Can you work these out from the model? Positions are in its coordinate system, mm. A direction names the side the tool comes from. Round coordinates to 2 decimals unless told otherwise and drop trailing zeros. Order: outer loops, then holes, each group sorted by start corner. A loop starts at its lowest first (then second) coordinate and runs counter-clockwise, first axis right, second up. Notation, with made-up numbers: M 33,84.5 L 70,84.5 A26 cw 70,119.5 Z; hole C 55.5,1.25 d4. An arc over 180 degrees is marked long. One line per question, with ' | ' between items.
```python
from build123d import *

# Parameters (mm, degrees)
CUT_EXTRUDE_1_REACH             = 31.394
SKETCH_3_R                      = 2
CUT_EXTRUDE_1_DIRECTION_2_DEPTH = 30.393876913


with BuildPart() as part:
    # 草图2 → 旋转1 (revolve)
    with BuildSketch(Plane.XY):
        Polygon((0, 0), (-20, 0), (-20, 2), (-17.5, 2), (-17.5, 8), (0, 8), align=None)
    revolve(axis=Axis((0, 8, 0), (0, -1, 0)))

    # 草图3 → 切除-拉伸1 (cut, up to next)
    with BuildSketch(Plane(origin=(0, 8, 0), x_dir=(1, 0, 0), z_dir=(0, 1, 0)), mode=Mode.PRIVATE) as cut_extrude_1_sk1:
        with Locations((0, 15)):
            Circle(SKETCH_3_R)
    cut_extrude_1_tool1 = extrude(cut_extrude_1_sk1.sketch, amount=-CUT_EXTRUDE_1_REACH, mode=Mode.PRIVATE) & part.part
    # 草图3 → 切除-拉伸1 (cut, up to next)
    with BuildSketch(Plane(origin=(0, 8, 0), x_dir=(1, 0, 0), z_dir=(0, 1, 0)), mode=Mode.PRIVATE) as cut_extrude_1_sk2:
        with Locations((15, 0)):
            Circle(SKETCH_3_R)
    cut_extrude_1_tool2 = extrude(cut_extrude_1_sk2.sketch, amount=-CUT_EXTRUDE_1_REACH, mode=Mode.PRIVATE) & part.part
    # 草图3 → 切除-拉伸1 (cut, up to next)
    with BuildSketch(Plane(origin=(0, 8, 0), x_dir=(1, 0, 0), z_dir=(0, 1, 0)), mode=Mode.PRIVATE) as cut_extrude_1_sk3:
        with Locations((0, -15)):
            Circle(SKETCH_3_R)
    cut_extrude_1_tool3 = extrude(cut_extrude_1_sk3.sketch, amount=-CUT_EXTRUDE_1_REACH, mode=Mode.PRIVATE) & part.part
    # 草图3 → 切除-拉伸1 (cut, up to next)
    with BuildSketch(Plane(origin=(0, 8, 0), x_dir=(1, 0, 0), z_dir=(0, 1, 0)), mode=Mode.PRIVATE) as cut_extrude_1_sk4:
        with Locations((-15, 0)):
            Circle(SKETCH_3_R)
    cut_extrude_1_tool4 = extrude(cut_extrude_1_sk4.sketch, amount=-CUT_EXTRUDE_1_REACH, mode=Mode.PRIVATE) & part.part
    add(cut_extrude_1_tool1.solids().sort_by_distance((0, 8, -15))[0], mode=Mode.SUBTRACT)
    add(cut_extrude_1_tool2.solids().sort_by_distance((15, 8, 0))[0], mode=Mode.SUBTRACT)
    add(cut_extrude_1_tool3.solids().sort_by_distance((0, 8, 15))[0], mode=Mode.SUBTRACT)
    add(cut_extrude_1_tool4.solids().sort_by_distance((-15, 8, 0))[0], mode=Mode.SUBTRACT)

    # 草图3 → 切除-拉伸1 direction 2 (cut)
    with BuildSketch(Plane(origin=(0, 8, 0), x_dir=(1, 0, 0), z_dir=(0, 1, 0))):
        with Locations((0, 15)):
            Circle(SKETCH_3_R)
        with Locations((15, 0)):
            Circle(SKETCH_3_R)
        with Locations((0, -15)):
            Circle(SKETCH_3_R)
        with Locations((-15, 0)):
            Circle(SKETCH_3_R)
    extrude(amount=CUT_EXTRUDE_1_DIRECTION_2_DEPTH, mode=Mode.SUBTRACT)


solid = part.part
```
(1) Will these pins go through, and if not, where does the flat tip stop? pin 1 Ø1 at (x, y) = (-3.5, 4.5) entering from +Z; pin 2 Ø1.5 at (x, y) = (-15, 2.5) entering from -Z; pin 3 Ø2 at (x, y) = (16, 4.5) entering from +Z.
Final values:
pin 1: z = 17.24 | pin 2: z = -13.84 | pin 3: z = 9.01
(2) If we section it at B-B on x = 0: Please give me the cut outline in (y, z).
Final values:
outline: M 0,-20 L 2,-20 L 2,-17.5 L 8,-17.5 L 8,-17 L 0,-17 Z; M 0,-13 L 8,-13 L 8,13 L 0,13 Z; M 0,17 L 8,17 L 8,17.5 L 2,17.5 L 2,20 L 0,20 Z
(3) If we section it at A-A on z = 0: Please give me the cut outline in (x, y).
Final values:
outline: M -20,0 L -17,0 L -17,8 L -17.5,8 L -17.5,2 L -20,2 Z; M -13,0 L 13,0 L 13,8 L -13,8 Z; M 17,0 L 20,0 L 20,2 L 17.5,2 L 17.5,8 L 17,8 Z
(4) Thinking about a two-plate mould opening in Z: for faces 3 (the cylindrical face through (13.4, 4.1, 1.2)), 4 (the cylindrical face through (13.887, 5.042, 10.648)), 5 (the flat face through (0, 8, 0)), which applies, released by +Z, released by -Z, zero draft, split by the parting line, or undercut?
Final values:
face 3: undercut | face 4: split by the parting line | face 5: zero draft
(5) If we section it at D-D on x = 15: Please give me the cut outline in (y, z), plus the area to 3 significant figures.
Final values:
outline: M 0,-13.23 L 2,-13.23 L 2,-9.01 L 8,-9.01 L 8,-2 L 0,-2 Z; M 0,2 L 8,2 L 8,9.01 L 2,9.01 L 2,13.23 L 0,13.23 Z | area: 129 mm^2
(6) If we section it at C-C on y = 1: Please give me the cut outline in (x, z).
Final values:
outline: C 0,0 d40; hole C -15,0 d4; hole C 0,-15 d4; hole C 0,15 d4; hole C 15,0 d4
(7) Please list where these lines run through material, in increasing order: probe 1 along Z at (x, y) = (0, 5); probe 2 along Z at (x, y) = (1.5, 4.75). Write a range as [from, to].
Final values:
probe 1: [-17.5, -17], [-13, 13], [17, 17.5] | probe 2: [-17.44, -16.32], [-13.68, 13.68], [16.32, 17.44]
(8) On a 3-axis mill with a long thin cutter (end or side, diameter ignored), from which of +Z, -Z, +X, -X, +Y, -Y can I reach the whole of each face in a straight line? I mean faces 1 (the cylindrical face through (0, 4, 13)), 2 (the flat face through (0, 2, 18)). Say none if no direction works.
Final values:
face 1: +Y, -Y | face 2: +Y
